Input: part model. Units: mm. Frame: model coordinates. Face numbers are marked on the shaded views. Round coordinates to 2 decimals unless told otherwise and drop trailing zeros. Order: outer loops, then holes, each group sorted by start corner. A loop starts at its lowest first (then second) coordinate and runs counter-clockwise, first axis right, second up.
Item 1: First-contact query: pin 1 (2 mm diameter, centred on x = 10, z = -25, fed in from -Y); pin 2 (0.9 mm diameter, centred on y = 2, z = -15, fed in from -X). Flat tips, straight axial feed; report the tip coordinate or a pass-through.
Item 2: Cut plane C-C on y = 4.1. Output: boundary loops of the cut face in (x, z).
Item 3: Cut plane B-B on x = 10. Output: boundary loops of the cut face in (y, z), then the cut area to 3 significant figures.
Item 4: Line query: L1, parallel to X at y = 1.85, z = -5; L2, parallel to Z at x = 9.5, y = 0.4; L3, parallel to Z at x = 2.75, y = 2.9. Output: solid intervals per line, ascending.
Item 5: Cut plane A-A on z = -15. Output: boundary loops of the cut face in (x, y).
Item 6: Cut plane D-D on y = 1.25. Output: boundary loops of the cut face in (x, z).
Item 7: Mould query, pull axis Z, two halves, no side actions, for the marked faces 1, 2, 3 and 4. Classes: released by +Z, released by -Z, zero draft, split by the parting line, or undercut.
```python
from build123d import *

# Parameters (mm, degrees)
SKETCH1_W           = 20
SKETCH1_H           = 30
BOSS_EXTRUDE1_DEPTH = 5
CUT_EXTRUDE1_DEPTH  = 8
SKETCH3_R           = 1.75
CUT_EXTRUDE2_DEPTH  = 37.400549446
SKETCH4_W           = 5.7
SKETCH4_H           = 3
CUT_EXTRUDE3_DEPTH  = 18


with BuildPart() as part:
    # Sketch1 → Boss-Extrude1 (new body)
    with BuildSketch(Plane(origin=(0, 0, 0), x_dir=(1, 0, 0), z_dir=(0, 1, 0))):
        with Locations((10, 15)):
            Rectangle(SKETCH1_W, SKETCH1_H)
    extrude(amount=BOSS_EXTRUDE1_DEPTH)

    # Sketch2 → Cut-Extrude1 (cut)
    with BuildSketch(Plane(origin=(0, 5, 0), x_dir=(1, 0, 0), z_dir=(0, 1, 0))):
        with BuildLine():
            Line((5, 16.75), (15, 16.75))
            ThreePointArc((15, 16.75), (16.75, 15), (15, 13.25))
            Line((15, 13.25), (5, 13.25))
            ThreePointArc((5, 13.25), (3.25, 15), (5, 16.75))
        make_face()
    extrude(amount=-CUT_EXTRUDE1_DEPTH, mode=Mode.SUBTRACT)

    # Sketch3 → Cut-Extrude2 (cut, through all)
    with BuildSketch(Plane(origin=(0, 5, 0), x_dir=(1, 0, 0), z_dir=(0, 1, 0))):
        with Locations(Location((10, 25, 0), (0, 0, 270))):
            Circle(SKETCH3_R)
        with Locations(Location((10, 5, 0), (0, 0, 270))):
            Circle(SKETCH3_R)
    extrude(amount=-CUT_EXTRUDE2_DEPTH, mode=Mode.SUBTRACT)

    # Sketch4 → Cut-Extrude3 (cut)
    with BuildSketch(Plane.ZY):
        with Locations((-15.15, 1.5)):
            Rectangle(SKETCH4_W, SKETCH4_H)
    extrude(amount=-CUT_EXTRUDE3_DEPTH, mode=Mode.SUBTRACT)


solid = part.part
```
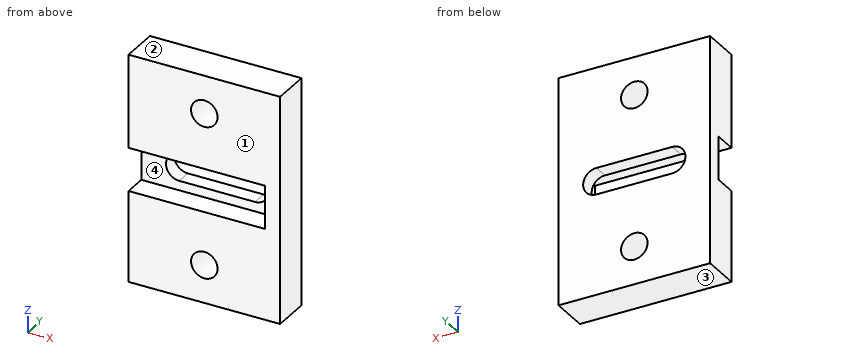
From the geometry:
1. pin 1: passes through
1. pin 2: stops at x = 18
2. outline: (0, -30) - (20, -30) - (20, 0) - (0, 0) - close; hole (5, -16.75) - (15, -16.75) arc R1.75 ccw to (15, -13.25) - (5, -13.25) arc R1.75 ccw to start; hole circle Ø3.5 at (10, -25); hole circle Ø3.5 at (10, -5)
3. outline: (0, -30) - (5, -30) - (5, -26.75) - (0, -26.75) - close; (0, -23.25) - (5, -23.25) - (5, -16.75) - (3, -16.75) - (3, -18) - (0, -18) - close; (0, -12.3) - (3, -12.3) - (3, -13.25) - (5, -13.25) - (5, -6.75) - (0, -6.75) - close; (0, -3.25) - (5, -3.25) - (5, 0) - (0, 0) - close
3. area: 90.9 mm2
4. L1: x = 0 to 8.25, 11.75 to 20
4. L2: z = -30 to -26.68, -23.32 to -18, -12.3 to -6.68, -3.32 to 0
4. L3: z = -30 to -18, -12.3 to 0
5. outline: (0, 3) - (3.25, 3) - (3.25, 5) - (0, 5) - close; (16.75, 3) - (18, 3) - (18, 0) - (20, 0) - (20, 5) - (16.75, 5) - close
6. outline: (0, -30) - (20, -30) - (20, 0) - (0, 0) - (0, -12.3) - (18, -12.3) - (18, -18) - (0, -18) - close; hole circle Ø3.5 at (10, -25); hole circle Ø3.5 at (10, -5)
7. face 1: zero draft
7. face 2: released by +Z
7. face 3: released by -Z
7. face 4: undercut
